The figure shows three views and two pictorial views of one solid part (mm, origin at its lowest corner). Answer the questions. A direction names the side the tool comes from. Give positions to 0.01 mm unless a question says otherwise; leave off trailing zeros. Loops run counter-clockwise (first coordinate to the right, second up) from the corner with the lowest first, then second, coordinate; pieces in that order, holes last. Notation, with made-up numbers: (-1.5, 44) - (20.5, 44) arc R18 ccw to (20.5, 64) - close; hole circle Ø5 at (-39, 40.25). An arc over 180 degrees is marked (long way). One line per question, with ' | ' between items.
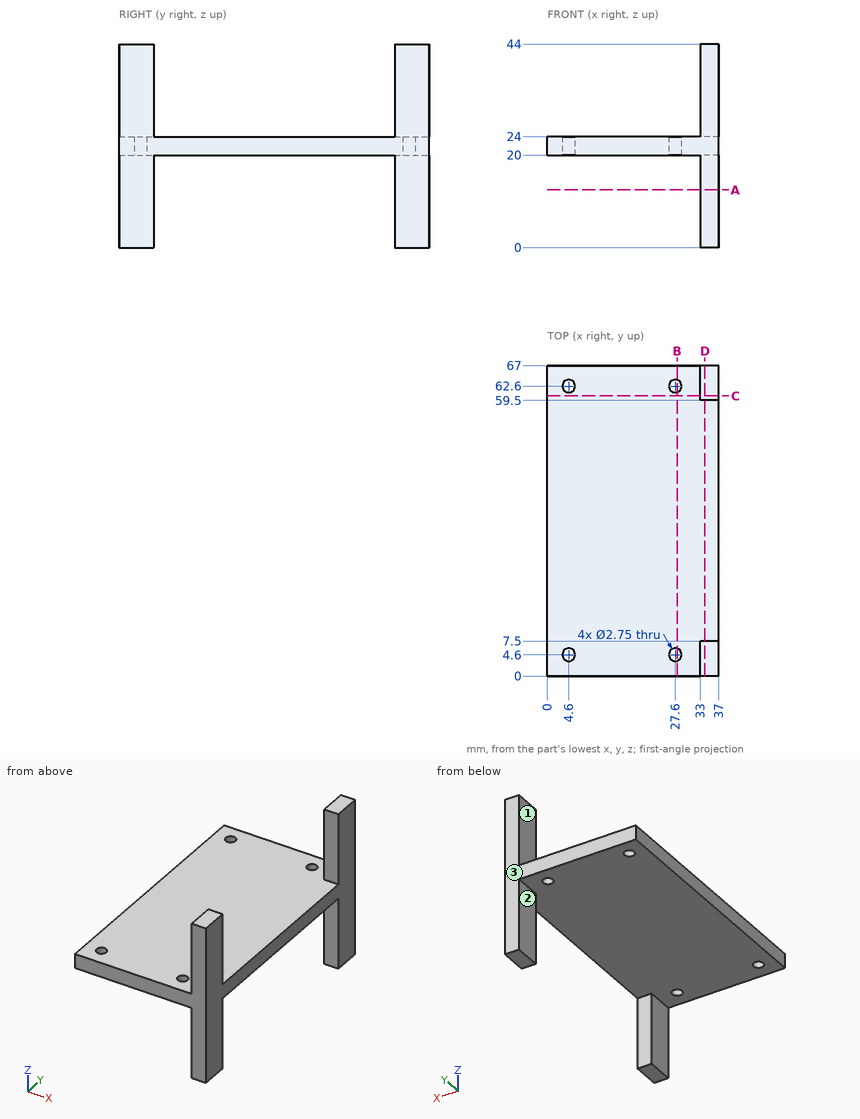
1. Flat-ended cylindrical pins translate along their axes: pin 1 (1 mm diameter, centred on x = 24, y = 59.5, fed in from +Z); pin 2 (2 mm diameter, centred on y = 64, z = 34.5, fed in from -X); pin 3 (4.5 mm diameter, centred on x = 4.6, y = 4.6, fed in from -Z). Find the tip coordinate at first contact, or state that the pin passes through.
Evaluation:
pin 1: z = 24 | pin 2: x = 33 | pin 3: z = 20
2. Which of the six approach directions +Z, -Z, +X, -X, +Y, -Y give full straight-line access (tool end or side, diameter ignored) to the marked faces 1, 2 and 3?
Evaluation:
face 1: +Z, -X, +Y, -Y | face 2: -Z, -X, +Y, -Y | face 3: +Z, -Z, +X, -X, +Y
3. Find section A-A on z = 12.5. Write down the section's boundary in (x, y), then the cut area to 3 significant figures.
Evaluation:
outline: (33, 0) - (37, 0) - (37, 7.5) - (33, 7.5) - close; (33, 59.5) - (37, 59.5) - (37, 67) - (33, 67) - close | area: 60.0 mm2
4. Find section B-B on x = 28. Write down the section's boundary in (y, z), then the cut area to 3 significant figures.
Evaluation:
outline: (0, 20) - (3.28, 20) - (3.28, 24) - (0, 24) - close; (5.92, 20) - (61.28, 20) - (61.28, 24) - (5.92, 24) - close; (63.92, 20) - (67, 20) - (67, 24) - (63.92, 24) - close | area: 247 mm2
5. Find section D-D on x = 34. Write down the section's boundary in (y, z), then the cut area to 3 significant figures.
Evaluation:
outline: (0, 0) - (7.5, 0) - (7.5, 20) - (59.5, 20) - (59.5, 0) - (67, 0) - (67, 44) - (59.5, 44) - (59.5, 24) - (7.5, 24) - (7.5, 44) - (0, 44) - close | area: 868 mm2
6. Find section C-C on y = 60.5. Write down the section's boundary in (x, z).
Evaluation:
outline: (0, 20) - (33, 20) - (33, 0) - (37, 0) - (37, 44) - (33, 44) - (33, 24) - (0, 24) - close
7. Consider L1, parallel to Y at x = 35.5, z = 11; L2, parallel to Z at x = 23.5, y = 58.5. Determine where each line is inside the solid, lowest interval first.
Evaluation:
L1: 0 to 7.5, 59.5 to 67 | L2: 20 to 24
